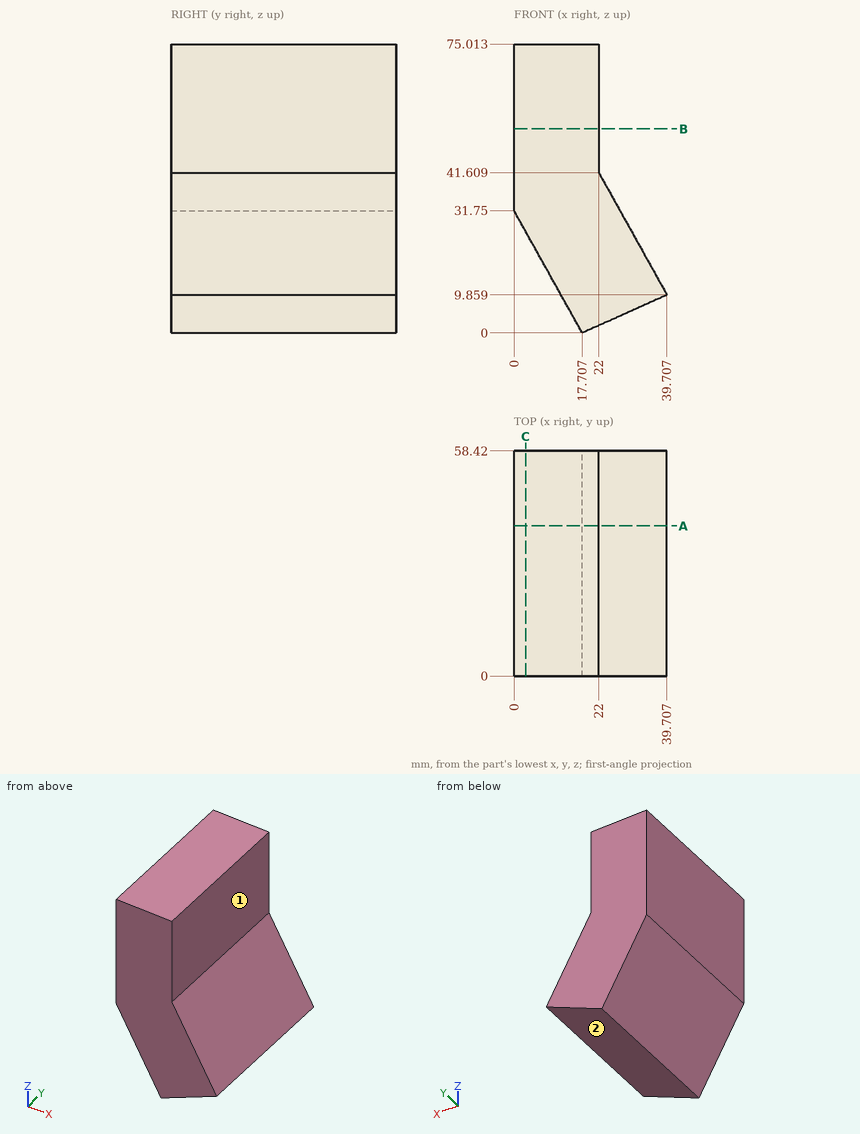
Here's the drawing with two shaded views (mm, measured from the low corner). I have some questions. A direction names the side the tool comes from. Coordinates: 2 decimals unless noted, no trailing zeros. Order: outer loops, then holes, each group sorted by start corner. A loop starts at its lowest first (then second) coordinate and runs counter-clockwise, first axis right, second up. Notation, with made-up numbers: M 43.25,0 L 47.25,0 A12 ccw 47.25,22 Z; hole C 24,36 d11. An arc over 180 degrees is marked long. Write item = value, one per line.
(1) Suppose I cut it at A-A on y = 39. Please give me the cut outline in (x, z).
Results are:
outline = M 0,31.75 L 17.71,0 L 39.71,9.86 L 22,41.61 L 22,75.01 L 0,75.01 Z
(2) For the marked faces 1 and 2, which set-ups out of +Z, -Z, +X, -X, +Y, -Y let a thin tool reach every point of the face, with its end or its side?
Results are:
face_1 = +Z, +X, +Y, -Y
face_2 = -Z, +X, +Y, -Y
(3) Suppose I cut it at C-C on x = 3. Please give me the cut outline in (y, z), plus the area to 3 significant figures.
Results are:
outline = M 0,26.37 L 58.42,26.37 L 58.42,75.01 L 0,75.01 Z
area = 2,840 mm2
(4) Suppose I cut it at B-B on z = 53. Please give me the cut outline in (x, y).
Results are:
outline = M 0,0 L 22,0 L 22,58.42 L 0,58.42 Z
(5) I need wall thicknesses on line 1 along X through (y, z) = (8, 60.5); line 2 along Z through (x, y) = (37, 41) (1 decimal); line 3 along Z through (x, y) = (9, 45) (1 decimal). Which ranges of each line are inside material? Lowest first, please. Write a range as [from, to].
Results are:
line_1 = [0, 22]
line_2 = [8.6, 14.7]
line_3 = [15.6, 75]
(6) For pin 1 Ø12 at (y, z) = (17, 15.5) entering from -X; pin 2 Ø4 at (y, z) = (20, 12.5) entering from +X; pin 3 Ø3 at (x, z) = (17, 25) entering from -Y; pin 4 Ø8 at (y, z) = (34.5, 63.5) entering from +X, each with a flat end and sliding along its axis, tell me the tip position at first contact or that it passes through.
Results are:
pin_1 = 5.72
pin_2 = 39.35
pin_3 = 0
pin_4 = 22
